Can you work these out from the model? Positions are in its coordinate system, mm. Face numbers are marked on the shaded views. A direction names the side the tool comes from. Give positions to 0.01 mm unless a question says otherwise; leave off trailing zeros. Write each loop counter-clockwise with the first axis right and the second up, starting at its lowest first coordinate (ties: lowest second). Pieces come first, ordered by that corner, then holes.
Autodesk Inventor part; units mm, degrees
ref_plane "YZ Plane" through (0, 0, 0) normal (1, 0, 0) x (0, 1, 0)
ref_plane "XZ Plane" through (0, 0, 0) normal (0, 1, 0) x (-1, 0, 0)
ref_plane "XY Plane" through (0, 0, 0) normal (0, 0, 1) x (1, 0, 0)
ref_plane "Work Plane1" through (0, 0, 0) normal (0, 0, 1) x (1, 0, 0)
sketch "Sketch1" plane through (0, 0, 0) normal (0, 0, 1) x (1, 0, 0)
  circle A0 centre (-70.0994, -13.8265) radius 7.5
  circle A1 centre (69.9006, -13.8265) radius 7.5
  circle A2 centre (-0.0994, -13.8265) radius 5.08
  arc A3 (-82.5729, -11.3834) -> (-57.3889, -13.8265) centre (-70.0994, -13.8265) ccw
  line L0 (-57.3889, 5.8585) -> (-57.3889, -13.8265)
  line L1 (-54.2139, 9.0335) -> (-57.3889, 5.8585)
  line L2 (-25.4994, 9.0335) -> (-54.2139, 9.0335)
  arc A4 (-17.8794, 1.4135) -> (-25.4994, 9.0335) centre (-25.4994, 1.4135) ccw
  line L3 (-17.8794, -26.5265) -> (-17.8794, 1.4135)
  line L4 (17.6806, -26.5265) -> (-17.8794, -26.5265)
  line L5 (17.6806, 1.4135) -> (17.6806, -26.5265)
  arc A5 (25.3006, 9.0335) -> (17.6806, 1.4135) centre (25.3006, 1.4135) ccw
  line L6 (54.0151, 9.0335) -> (25.3006, 9.0335)
  line L7 (57.1901, 5.8585) -> (54.0151, 9.0335)
  line L8 (57.1901, -13.8265) -> (57.1901, 5.8585)
  arc A6 (57.1901, -13.8265) -> (82.6111, -13.8265) centre (69.9006, -13.8265) ccw
  line L9 (79.9006, 14.1135) -> (82.6111, -13.8265)
  line L10 (-80.0994, 14.1135) -> (79.9006, 14.1135)
  line L11 (-82.5729, -11.3834) -> (-80.0994, 14.1135)
  line L12 (-25.4994, 9.0335) -> (25.3006, 9.0335)
  point P0 (0, 0)
extrude "Extrusion1" add sketch "Sketch1" against normal blind 25.4 contours L11 L10 L9 A6 L8 L7 L6 L12 L2 L1 L0 A3
sketch "Sketch2" plane through (0, 0, 0) normal (0, 0, 1) x (1, 0, 0)
  circle A0 centre (69.9006, -13.8265) radius 7.5
  circle A1 centre (-70.0994, -13.8265) radius 7.5
  line L0 (-57.3889, -13.8265) -> (-57.3889, 5.8585)
  line L1 (-57.3889, 5.8585) -> (-54.2139, 9.0335)
  line L2 (-54.2139, 9.0335) -> (54.0151, 9.0335)
  line L3 (54.0151, 9.0335) -> (57.1901, 5.8585)
  line L4 (57.1901, 5.8585) -> (57.1901, -13.8265)
  arc A2 (57.1901, -13.8265) -> (82.6111, -13.8265) centre (69.9006, -13.8265) ccw
  line L5 (82.6111, -13.8265) -> (79.9006, 14.1135)
  line L6 (79.9006, 14.1135) -> (-80.0994, 14.1135)
  line L7 (-80.0994, 14.1135) -> (-82.5729, -11.3834)
  arc A3 (-82.5729, -11.3834) -> (-57.3889, -13.8265) centre (-70.0994, -13.8265) ccw
  circle A4 centre (-70.0994, -13.8265) radius 5
  circle A5 centre (69.9006, -13.8265) radius 5
  point P0 (0, 0)
  dimension "d2" = 10
  dimension "d3" = 10
extrude "Extrusion2" add sketch "Sketch2" against normal blind 1 contours A0 | A1
sketch "Sketch3" plane through (-54.2139, 9.0335, 0) normal (0, -1, 0) x (1, 0, 0)
  line L0 (0, 0) -> (108.229, 0)
  line L1 (108.229, -25.4) -> (0, -25.4)
  line L2 (-11.8855, 142.225) -> (-11.8855, -175.0375)
  line L3 (-25.8855, -146.05) -> (-25.8855, 93.95)
  line L4 (-25.8855, 0) -> (-25.8855, -25.4)
  line L5 (-25.8855, -12.7) -> (4.1145, -12.7)
  circle A0 centre (4.1145, -12.7) radius 2
  circle A1 centre (24.1145, -12.7) radius 2
  circle A2 centre (44.1145, -12.7) radius 2
  line L6 (54.2139, 0) -> (54.2139, -3.82)
  line L7 (134.3133, -12.7) -> (104.3133, -12.7)
  circle A3 centre (104.3133, -12.7) radius 2
  circle A4 centre (84.3133, -12.7) radius 2
  circle A5 centre (64.3133, -12.7) radius 2
  dimension "d6" = 30
  dimension "d9" = 4
  dimension "d10" = 4
  dimension "d11" = 4
extrude "Extrusion3" cut sketch "Sketch3" against normal blind 508
sketch "Sketch4" plane through (0, 0, 0) normal (0, 0, 1) x (1, 0, 0)
  circle A0 centre (69.9006, -13.8265) radius 5
  circle A1 centre (-70.0994, -13.8265) radius 5
  line L0 (-57.3889, -13.8265) -> (-57.3889, 5.8585)
  line L1 (-57.3889, 5.8585) -> (-54.2139, 9.0335)
  line L2 (-54.2139, 9.0335) -> (54.0151, 9.0335)
  line L3 (54.0151, 9.0335) -> (57.1901, 5.8585)
  line L4 (57.1901, 5.8585) -> (57.1901, -13.8265)
  arc A2 (57.1901, -13.8265) -> (82.6111, -13.8265) centre (69.9006, -13.8265) ccw
  line L5 (82.6111, -13.8265) -> (79.9006, 14.1135)
  line L6 (79.9006, 14.1135) -> (-80.0994, 14.1135)
  line L7 (-80.0994, 14.1135) -> (-82.5729, -11.3834)
  arc A3 (-82.5729, -11.3834) -> (-57.3889, -13.8265) centre (-70.0994, -13.8265) ccw
  line L8 (-57.3889, -13.8265) -> (-22.2837, 9.0335)
  line L9 (54.0151, 9.0335) -> (-54.2139, 9.0335)
  line L10 (-0.0994, 9.0335) -> (-0.0994, 6.3526)
  line L11 (-57.3889, 5.8585) -> (-57.3889, -13.8265)
  line L12 (-57.3889, -13.8265) -> (-57.3889, 9.0335)
  line L13 (-57.3889, 9.0335) -> (-22.2837, 9.0335)
  line L14 (57.1901, -13.8265) -> (57.1901, 5.8585)
  line L15 (54.0151, 9.0335) -> (-54.2139, 9.0335)
  line L16 (57.1901, -13.8265) -> (22.0849, 9.0335)
  line L17 (57.1901, -13.8265) -> (57.1901, 9.0335)
  line L18 (57.1901, 9.0335) -> (22.0849, 9.0335)
  point P0 (0, 0)
extrude "Extrusion4" add sketch "Sketch4" against normal blind 5.08 contours L0 L1 L2 L8 | L2 L3 L4 L16 | L18 L17 L3
properties part number "Bed"
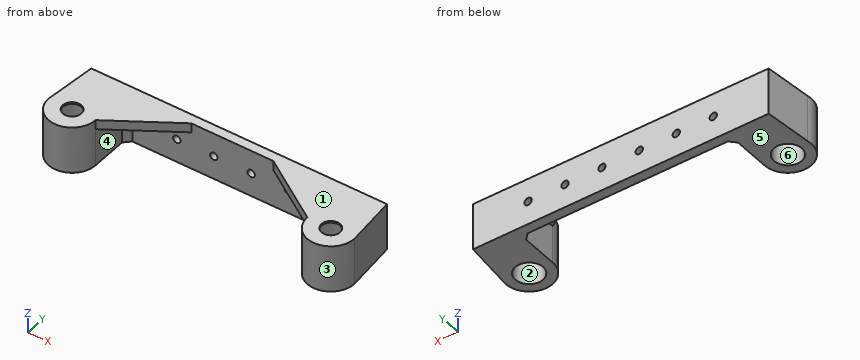
1) For the marked faces 4, 5 and 6, which set-ups out of +Z, -Z, +X, -X, +Y, -Y let a thin tool reach every point of the face, with its end or its side?
Values follow:
face 4: -Z, -Y
face 5: -Z, +X, -X, +Y, -Y
face 6: -Z
2) If we mould it in two halves opening along Y, with no side actions, what happens to the marked faces 1, 2 and 3? For each: +Y half, -Y half, draft (parallel to the pull), parting line (faces both ways), or undercut.
Values follow:
face 1: draft
face 2: undercut
face 3: -Y half
3) Please list where these lines run through material, in increasing order: L1, parallel to X at y = -18, z = -12; L2, parallel to Y at x = 7.5, z = -9; L3, parallel to X at y = -10.5, z = -21.5.
Values follow:
L1: x = -82.11 to -76.33, -63.87 to -58.09, 57.89 to 63.67, 76.13 to 81.91
L2: y = 9.03 to 14.11
L3: x = -82.49 to -76.82, -63.38 to -57.39, 57.19 to 63.18, 76.62 to 82.29
4) Suppose I cut it at B-B on z = -12.7. State how many separate pieces and enclosed holes the cut face has, plus the area to 3 significant figures.
Values follow:
separate pieces: 7
enclosed holes: 2
area: 1,970 mm2
5) For pin 1 Ø7.5 at (x, z) = (-24.5, -12) entering from -Y; pin 2 Ø1.5 at (x, y) = (-19.5, 8) entering from -Z; pin 3 Ø18.5 at (x, y) = (-43.5, -6.5) entering from -Z; pin 4 Ø6 at (y, z) = (-2.5, -20) entering from -X, each with a flat end and sliding along its axis, tell me the tip position at first contact or that it passes through.
Values follow:
pin 1: stops at y = 9.03
pin 2: passes through
pin 3: stops at z = -5.08
pin 4: stops at x = -82
6) Suppose I cut it at C-C on y = -23. Write out the boundary of the cut face in (x, z).
Values follow:
outline: (-78.9, -25.4) - (-61.3, -25.4) - (-61.3, 0) - (-78.9, 0) - close; (61.1, -25.4) - (78.7, -25.4) - (78.7, 0) - (61.1, 0) - close
7) Suppose I cut it at D-D on x = -73. Write out the boundary of the cut face in (y, z), plus the area to 3 significant figures.
Values follow:
outline: (-26.2, -25.4) - (-20.74, -25.4) - (-20.74, -1) - (-17.9, -1) - (-17.9, 0) - (-26.2, 0) - close; (-9.75, -1) - (-6.91, -1) - (-6.91, -25.4) - (14.11, -25.4) - (14.11, 0) - (-9.75, 0) - close
area: 678 mm2
8) Suppose I cut it at A-A on z = -20. Write out the boundary of the cut face in (x, y).
Values follow:
outline: (-82.57, -11.38) arc R12.71 ccw (long way) to (-57.39, -13.83) - (-57.39, 5.86) - (-54.21, 9.03) - (54.02, 9.03) - (57.19, 5.86) - (57.19, -13.83) arc R12.71 ccw to (82.61, -13.83) - (79.9, 14.11) - (-80.1, 14.11) - close; hole circle Ø15 at (-70.1, -13.83); hole circle Ø15 at (69.9, -13.83)
